from build123d import *

# Parameters (mm, degrees)
BOSS_EXTRUDE1_DEPTH                  = 444.5
F_10_32_TAPPED_HOLE1_D               = 4.0386
F_10_32_TAPPED_HOLE1_DEPTH           = 15.07744
F_10_32_TAPPED_HOLE1_TIP             = 1.213317848
F_10_32_TAPPED_HOLE1_ON_FACE_2_D     = 4.0386
F_10_32_TAPPED_HOLE1_ON_FACE_2_DEPTH = 15.07744
F_10_32_TAPPED_HOLE1_ON_FACE_2_TIP   = 1.213317848


with BuildPart() as part:
    # Sketch1 → Boss-Extrude1 (new body)
    with BuildSketch(Plane.XY):
        with BuildLine():
            ThreePointArc((6.35, 2.590301913), (5.939202219, 3.429), (5.41826726, 4.204110358))
            Line((5.41826726, 4.204110358), (0.93173274, 6.79441227))
            ThreePointArc((0.93173274, 6.79441227), (0, 6.858), (-0.93173274, 6.79441227))
            Line((-0.93173274, 6.79441227), (-5.41826726, 4.204110358))
            ThreePointArc((-5.41826726, 4.204110358), (-5.939202219, 3.429), (-6.35, 2.590301913))
            Line((-6.35, 2.590301913), (-6.35, -2.590301913))
            ThreePointArc((-6.35, -2.590301913), (-5.939202219, -3.429), (-5.41826726, -4.204110358))
            Line((-5.41826726, -4.204110358), (-0.93173274, -6.79441227))
            ThreePointArc((-0.93173274, -6.79441227), (0, -6.858), (0.93173274, -6.79441227))
            Line((0.93173274, -6.79441227), (5.41826726, -4.204110358))
            ThreePointArc((5.41826726, -4.204110358), (5.939202219, -3.429), (6.35, -2.590301913))
            Line((6.35, -2.590301913), (6.35, 2.590301913))
        make_face()
    extrude(amount=BOSS_EXTRUDE1_DEPTH)

    # #10-32 Tapped Hole1
    with Locations(Plane.XY.offset(444.5)):
        with Locations((0, 0)):
            Hole(F_10_32_TAPPED_HOLE1_D / 2, depth=F_10_32_TAPPED_HOLE1_DEPTH)
            with Locations((0, 0, -(F_10_32_TAPPED_HOLE1_DEPTH + F_10_32_TAPPED_HOLE1_TIP / 2))):  # 118° drill point
                Cone(0, F_10_32_TAPPED_HOLE1_D / 2, F_10_32_TAPPED_HOLE1_TIP, mode=Mode.SUBTRACT)

    # #10-32 Tapped Hole1 on face 2
    with Locations(Plane(origin=(0, 0, 0), x_dir=(-1, 0, 0), z_dir=(0, 0, -1))):
        with Locations((0, 0)):
            Hole(F_10_32_TAPPED_HOLE1_ON_FACE_2_D / 2, depth=F_10_32_TAPPED_HOLE1_ON_FACE_2_DEPTH)
            with Locations((0, 0, -(F_10_32_TAPPED_HOLE1_ON_FACE_2_DEPTH + F_10_32_TAPPED_HOLE1_ON_FACE_2_TIP / 2))):  # 118° drill point
                Cone(0, F_10_32_TAPPED_HOLE1_ON_FACE_2_D / 2, F_10_32_TAPPED_HOLE1_ON_FACE_2_TIP, mode=Mode.SUBTRACT)


solid = part.part
Could you check a few things on this model? Use its own coordinates, in mm. Coordinates: 2 decimals unless noted, no trailing zeros. Order: outer loops, then holes, each group sorted by start corner. A loop starts at its lowest first (then second) coordinate and runs counter-clockwise, first axis right, second up.
Q1. Will these pins go through, and if not, where does the flat tip stop? pin 1 (1.5 mm diameter, centred on x = 0.5, y = 0, fed in from +Z); pin 2 (3 mm diameter, centred on x = -5, z = 54.5, fed in from -Y).
Q2. Suppose I cut it at A-A on z = 86. Please give me the cut outline in (x, y), and give its area (3 significant figures).
Q3. Please list where these lines run through material, in increasing order: L1, parallel to Y at x = 0, z = 11; L2, parallel to X at y = 0, z = 11.25; L3, parallel to Y at x = 1, z = 27 (3 decimals).
Answer:
1. pin 1: stops at z = 428.96
1. pin 2: stops at y = -5.31
2. outline: (-6.35, -2.59) arc R6.86 ccw to (-5.42, -4.2) - (-0.93, -6.79) arc R6.86 ccw to (0.93, -6.79) - (5.42, -4.2) arc R6.86 ccw to (6.35, -2.59) - (6.35, 2.59) arc R6.86 ccw to (5.42, 4.2) - (0.93, 6.79) arc R6.86 ccw to (-0.93, 6.79) - (-5.42, 4.2) arc R6.86 ccw to (-6.35, 2.59) - close
2. area: 137 mm2
3. L1: y = -6.86 to -2.02, 2.02 to 6.86
3. L2: x = -6.35 to -2.02, 2.02 to 6.35
3. L3: y = -6.755 to 6.755
